Design review of the part built by this model. Coordinates are the model's own, in mm. Face numbers are marked on the shaded views. A direction names the side the tool comes from. Coordinates: 2 decimals unless noted, no trailing zeros. Loops run counter-clockwise (first coordinate to the right, second up) from the corner with the lowest first, then second, coordinate; pieces in that order, holes last. Notation, with made-up numbers: M 50,-9.75 L 87,-9.75 A20 ccw 87,-1.75 Z; hole C 17.25,10 d11. An arc over 180 degrees is marked long. Answer as CSV lines item,"result". Start each with the question number.
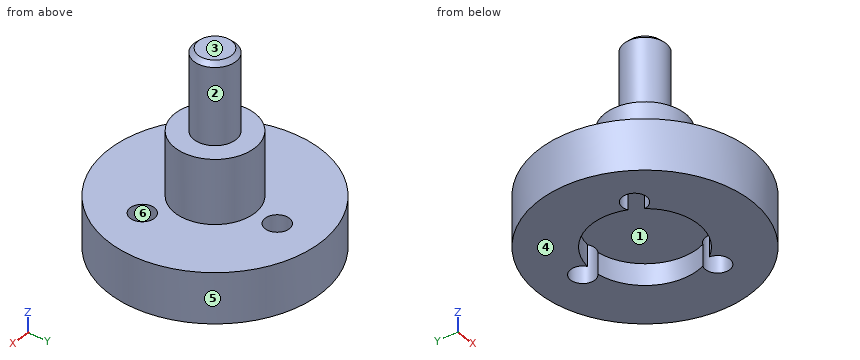
from build123d import *

# Parameters (mm, degrees)
SKETCH1_R                    = 12.7
MOUNTING_FLANGE_DEPTH        = 6
SKETCH3_R                    = 6.35
MOTOR_SHAFT_RELIEF_DEPTH     = 2.54
SKETCH4_R                    = 1.45
SCREW_CLEARANCE_HOLES_DEPTH  = 19.936208702
SKETCH2_R                    = 2.5
DRIVE_SHAFT_DEPTH            = 17.272
CHAMFER1_SIZE                = 0.508
SKETCH5_R                    = 4.7625
SHAFT_SUPPORT_SHOULDER_DEPTH = 7.62


with BuildPart() as part:
    # Sketch1 → Mounting Flange (new body)
    with BuildSketch(Plane.XY):
        Circle(SKETCH1_R)
    extrude(amount=MOUNTING_FLANGE_DEPTH)

    # Sketch3 → Motor Shaft Relief (cut)
    with BuildSketch(Plane(origin=(0, 0, 0), x_dir=(-1, 0, 0), z_dir=(0, 0, -1))):
        Circle(SKETCH3_R)
    extrude(amount=-MOTOR_SHAFT_RELIEF_DEPTH, mode=Mode.SUBTRACT)

    # Sketch4 → Screw Clearance Holes (cut, through all)
    with BuildSketch(Plane.XY.offset(6)):
        with Locations((0, 7.5)):
            Circle(SKETCH4_R)
        with Locations((6.495190528, -3.75)):
            Circle(SKETCH4_R)
        with Locations((-6.495190528, -3.75)):
            Circle(SKETCH4_R)
    extrude(amount=-SCREW_CLEARANCE_HOLES_DEPTH, mode=Mode.SUBTRACT)

    # Sketch2 → Drive Shaft (add)
    with BuildSketch(Plane.XY.offset(6)):
        Circle(SKETCH2_R)
    extrude(amount=DRIVE_SHAFT_DEPTH)

    # Chamfer1
    chamfer1_edges = [part.edges().sort_by_distance(p)[0] for p in [
        (-2.5, 0, 23.272),
    ]]
    chamfer(chamfer1_edges, length=CHAMFER1_SIZE)

    # Sketch5 → Shaft Support Shoulder (add)
    with BuildSketch(Plane.XY.offset(6)):
        with Locations(Location((0, 0, 0), (0, 0, 180))):
            Circle(SKETCH5_R)
    extrude(amount=SHAFT_SUPPORT_SHOULDER_DEPTH)


solid = part.part
Item 1: Add section D-D (y = 0). Give the boundary of the cut face in (x, z), plus the area to 3 significant figures.
Item 2: Add section B-B (y = 7.5). Give the boundary of the cut face in (x, z).
Item 3: For pin 1 (2 mm diameter, centred on x = 6, y = -4, fed in from +Z); pin 2 (8 mm diameter, centred on x = -4.5, y = -3.5, fed in from +Z); pin 3 (4 mm diameter, centred on y = -2.5, z = 12, fed in from +X); pin 4 (12 mm diameter, centred on x = 0.5, z = 14, fed in from +Y), all flat-tipped, find the tip position at first contact; note any pin that passes through.
Item 4: Add section C-C (y = -3.25). Give the boundary of the cut face in (x, z), plus the area to 3 significant figures.
Item 5: Mouldability with a two-part tool opening along Y and no side actions: class the marked faces 4, 5 and 6 as released by +Y, released by -Y, zero draft, split by the parting line, or undercut.
Item 6: For the marked faces 1, 2 and 3, list the 3-axis set-ups (+Z, -Z, +X, -X, +Y, -Y) from which the entire face can be reached by the end or side of a thin tool; tool diameter is ignored.
Item 7: For line 1 along X through (y, z) = (-4, 3.75); line 2 along Z through (x, y) = (-6.5, 5.25); line 3 along Y through (x, z) = (-1.5, 17), list the stretches that pass through material, from the lowest coordinate up. Write a range as from..to.
Item 8: Add section A-A (x = 0). Give the boundary of the cut face in (y, z).
Response:
1,outline,"M -12.7,0 L -6.35,0 L -6.35,2.54 L 6.35,2.54 L 6.35,0 L 12.7,0 L 12.7,6 L 4.76,6 L 4.76,13.62 L 2.5,13.62 L 2.5,22.76 L 1.99,23.27 L -1.99,23.27 L -2.5,22.76 L -2.5,13.62 L -4.76,13.62 L -4.76,6 L -12.7,6 Z"
1,area,"241 mm²"
2,outline,"M -10.25,0 L -1.45,0 L -1.45,6 L -10.25,6 Z; M 1.45,0 L 10.25,0 L 10.25,6 L 1.45,6 Z"
3,pin 1,"z = 6"
3,pin 2,"z = 23.27"
3,pin 3,"x = 4.74"
3,pin 4,"y = 4.76"
4,outline,"M -12.28,0 L -7.86,0 L -7.86,6 L -12.28,6 Z; M -5.13,2.54 L 5.13,2.54 L 5.13,6 L 3.48,6 L 3.48,13.62 L -3.48,13.62 L -3.48,6 L -5.13,6 Z; M 7.86,0 L 12.28,0 L 12.28,6 L 7.86,6 Z"
4,area,"142 mm²"
5,face 4,"zero draft"
5,face 5,"split by the parting line"
5,face 6,"undercut"
6,face 1,"-Z"
6,face 2,"+Z"
6,face 3,"+Z, +X, -X, +Y, -Y"
7,line 1,"-12.05..-7.92, -5.07..5.07, 7.92..12.05"
7,line 2,"0..6"
7,line 3,"-2..2"
8,outline,"M -12.7,0 L -6.35,0 L -6.35,2.54 L 6.05,2.54 L 6.05,6 L 4.76,6 L 4.76,13.62 L 2.5,13.62 L 2.5,22.76 L 1.99,23.27 L -1.99,23.27 L -2.5,22.76 L -2.5,13.62 L -4.76,13.62 L -4.76,6 L -12.7,6 Z; M 8.95,0 L 12.7,0 L 12.7,6 L 8.95,6 Z"
